```python
from build123d import *

# Parameters (mm, degrees)
F0_R     = 7
F1_DEPTH = 8
F1_TAPER = -30
F2_R     = 6
F3_DEPTH = 3
F4_R     = 1.1
F5_DEPTH = 25


with BuildPart() as f1:
    # F0 (on Top) → F1 (new body)
    with BuildSketch(Plane.XY):
        Circle(F0_R)
    extrude(amount=F1_DEPTH, taper=F1_TAPER)

    # F2 (on face) → F3 (cut)
    with BuildSketch(Plane(origin=(0, 0, 0), x_dir=(1, 0, 0), z_dir=(0, 0, -1))):
        Circle(F2_R)
    extrude(amount=-F3_DEPTH, mode=Mode.SUBTRACT)

    # F4 (on face) → F5 (cut)
    with BuildSketch(Plane.XY.offset(8)):
        Circle(F4_R)
    extrude(amount=-F5_DEPTH, mode=Mode.SUBTRACT)


solid = f1.part
```
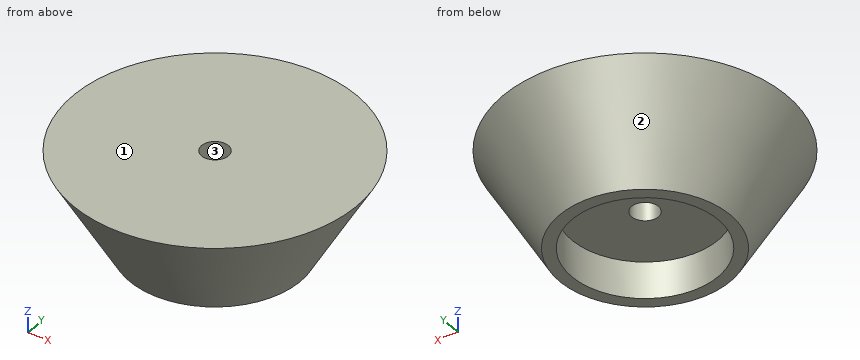
The listing builds one solid part. Answer for the finished solid, in the listing's coordinates (mm). Face numbers are marked on the shaded views. Round coordinates to 2 decimals unless told otherwise and drop trailing zeros. Loops run counter-clockwise (first coordinate to the right, second up) from the corner with the lowest first, then second, coordinate; pieces in that order, holes last.
Q1. Section C-C, the plane z = 6.5 is taken. Determine the outline of the cut face in (x, y).
Q2. Find the intervals of material crossed by line 1 (Z direction, x = 0.75, y = -4.75); line 2 (Y direction, x = 0.5, z = 5); line 3 (Y direction, x = -0.75, z = 3.5), in increasing order.
Q3. Given pin 1 Ø4 at (x, z) = (0.5, 5) entering from +Y; pin 2 Ø1.5 at (y, z) = (4, 3.5) entering from +X; pin 3 Ø11 at (x, y) = (0, 0) entering from -Z; pin 4 Ø2 at (x, y) = (0, 0) entering from -Z, each flat-ended and moving along its own axis, determine where each tip first touches the part or whether it passes through.
Q4. Section A-A, the plane x = 0 is taken. Determine the outline of the cut face in (y, z).
Q5. For a pull along X with two mould halves and no side action, classify the marked faces 1, 2 and 3 as released by +X, released by -X, zero draft, split by the parting line, or undercut.
Q6. Section B-B, the plane z = 2 is taken. Determine the outline of the cut face in (x, y), then the cut area to 3 significant figures.
Completed:
1. outline: circle Ø21.51 at (0, 0); hole circle Ø2.2 at (0, 0)
2. line 1: z = 3 to 8
2. line 2: y = -9.87 to -0.98, 0.98 to 9.87
2. line 3: y = -8.99 to -0.8, 0.8 to 8.99
3. pin 1: stops at y = 11.03
3. pin 2: stops at x = 8.67
3. pin 3: stops at z = 3
3. pin 4: passes through
4. outline: (-11.62, 8) - (-7, 0) - (-6, 0) - (-6, 3) - (-1.1, 3) - (-1.1, 8) - close; (1.1, 3) - (6, 3) - (6, 0) - (7, 0) - (11.62, 8) - (1.1, 8) - close
5. face 1: zero draft
5. face 2: split by the parting line
5. face 3: undercut
6. outline: circle Ø16.31 at (0, 0); hole circle Ø12 at (0, 0)
6. area: 95.8 mm2
